Input: part model. Units: mm. Frame: model coordinates. Face numbers are marked on the shaded views. Coordinates: 2 decimals unless noted, no trailing zeros. Write each loop counter-clockwise with the first axis right and the second up, starting at its lowest first coordinate (ties: lowest second). Pieces come first, ordered by that corner, then holes. Notation, with made-up numbers: (41.5, 82.5) -> (79.5, 82.5) arc R18 ccw to (79.5, 96.5) -> close; hole circle Ø10 at (22.5, 82.5). An arc over 180 degrees is marked (long way). Use one line per item in the form item = value. Start each with the question number.
(1) Cut plane C-C on z = -23.5. Return the cut outline in (x, y).
(2) Cut plane B-B on z = 0. Return the cut outline in (x, y).
(3) Cut plane A-A on x = 0. Return the cut outline in (y, z), plus the area to 3 significant figures.
(4) Pull-direction query (Z, two-part tool) for the marked faces 1 and 2; classes: released by +Z, released by -Z, zero draft, split by the parting line, or undercut.
(5) Cut plane D-D on y = 24. Return the cut outline in (x, z).
(6) First-contact query: pin 1 (1 mm diameter, centred on y = 51, z = 11, fed in from -X); pin 2 (8 mm diameter, centred on y = 20, z = 5.5, fed in from -X); pin 3 (3 mm diameter, centred on y = 37, z = 17, fed in from +X); pin 4 (3 mm diameter, centred on x = 22.5, z = -9.5, fed in from +Y). Flat tips, straight axial feed; report the tip coordinate or a pass-through.
(7) Ray query, line 1 along X through (y, z) = (14, 0); line 2 along Z through (x, y) = (19.5, 37). Return the intervals inside material, ascending.
```python
from build123d import *

# Parameters (mm, degrees)
SKETCH1_R           = 29.5
SKETCH1_R_2         = 27.5
BOSS_EXTRUDE1_DEPTH = 63
CUT_EXTRUDE1_DEPTH  = 33
CIRPATTERN1_COUNT   = 5


with BuildPart() as part:
    # Sketch1 → Boss-Extrude1 (new body)
    with BuildSketch(Plane(origin=(0, 0, 0), x_dir=(1, 0, 0), z_dir=(0, 1, 0))):
        with Locations(Location((0, 0, 0), (0, 0, 270))):
            Circle(SKETCH1_R)
        with Locations(Location((0, 0, 0), (0, 0, 270))):
            Circle(SKETCH1_R_2, mode=Mode.SUBTRACT)
    extrude(amount=BOSS_EXTRUDE1_DEPTH)

    # Sketch3 → Cut-Extrude1 (cut)
    with BuildSketch(Plane.XY):
        Polygon((0, 53), (12.5, 53), (12.5, 51), (-12.5, 51), (-12.5, 53), align=None)
    cut_extrude1 = extrude(amount=-CUT_EXTRUDE1_DEPTH, mode=Mode.SUBTRACT)

    # CirPattern1: Cut-Extrude1 ×5 about axis
    cirpattern1_axis = Axis((0, 0, 0), (0, 1, 0))
    for i in range(1, CIRPATTERN1_COUNT):
        add(cut_extrude1.rotate(cirpattern1_axis, i * 360 / CIRPATTERN1_COUNT), mode=Mode.SUBTRACT)


solid = part.part
```
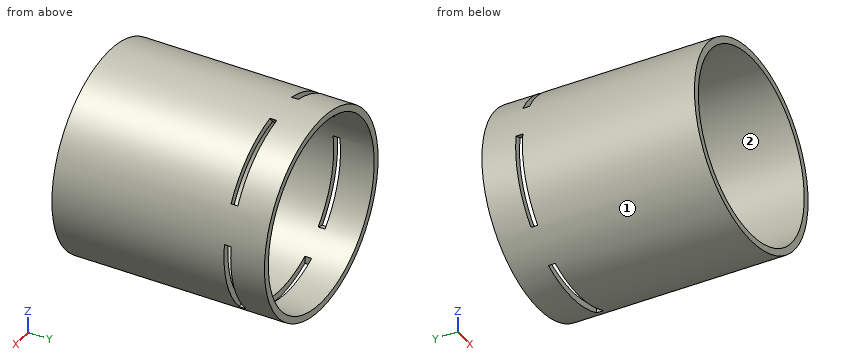
Values:
q1.outline = (-17.83, 0) -> (-14.28, 0) -> (-14.28, 63) -> (-17.83, 63) -> close; (14.28, 0) -> (17.83, 0) -> (17.83, 63) -> (14.28, 63) -> close
q2.outline = (-29.5, 0) -> (-27.5, 0) -> (-27.5, 51) -> (-29.5, 51) -> close; (-29.5, 53) -> (-27.5, 53) -> (-27.5, 63) -> (-29.5, 63) -> close; (27.5, 0) -> (29.5, 0) -> (29.5, 51) -> (27.5, 51) -> close; (27.5, 53) -> (29.5, 53) -> (29.5, 63) -> (27.5, 63) -> close
q3.outline = (0, -29.5) -> (51, -29.5) -> (51, -27.5) -> (0, -27.5) -> close; (0, 27.5) -> (63, 27.5) -> (63, 29.5) -> (0, 29.5) -> close; (53, -29.5) -> (63, -29.5) -> (63, -27.5) -> (53, -27.5) -> close
q3.area = 248 mm2
q4.face_1 = split by the parting line
q4.face_2 = undercut
q5.outline = circle Ø59 at (0, 0); hole circle Ø55 at (0, 0)
q6.pin_1 = -27.57
q6.pin_2 = -29.46
q6.pin_3 = 25.1
q6.pin_4 = through
q7.line_1 = -29.5 to -27.5, 27.5 to 29.5
q7.line_2 = -22.14 to -19.39, 19.39 to 22.14
